CAD build for the part. Positions are in the model's coordinates, mm. A direction names the side the tool comes from. Round coordinates to 2 decimals unless told otherwise and drop trailing zeros. Loops run counter-clockwise (first coordinate to the right, second up) from the corner with the lowest first, then second, coordinate; pieces in that order, holes last. Notation, with made-up numbers: M -10.5,-18 L 31.5,-18 A19 cw 31.5,6 Z; hole C 3,72.25 d1. An arc over 180 degrees is marked long. Use one line per item in the form item = value.
from build123d import *

# Parameters (mm, degrees)
SKETCH1_W           = 25
SKETCH1_H           = 30
BOSS_EXTRUDE1_DEPTH = 12
BOSS_EXTRUDE6_DEPTH = 12
CHAMFER1_SIZE       = 7
CHAMFER1_SIZE2      = 12.124355653
BOSS_EXTRUDE4_DEPTH = 12
SKETCH7_R           = 2.8
CUT_EXTRUDE2_DEPTH  = 12
CHAMFER2_SIZE       = 8
CHAMFER2_SIZE_2     = 14
CHAMFER3_SIZE       = 14
CHAMFER3_SIZE_2     = 8
FILLET2_R           = 20
FILLET3_R           = 1
FILLET4_R           = 1.5
SKETCH10_R          = 1
CUT_EXTRUDE3_DEPTH  = 41.859515416
SKETCH11_R          = 2
CUT_EXTRUDE4_DEPTH  = 41.859515416
SKETCH12_R          = 3.5
BOSS_EXTRUDE8_DEPTH = 2
FILLET5_R           = 3


with BuildPart() as part:
    # Sketch1 → Boss-Extrude1 (new body)
    with BuildSketch(Plane(origin=(0, 0, 0), x_dir=(1, 0, 0), z_dir=(0, 1, 0))):
        Rectangle(SKETCH1_W, SKETCH1_H)
        Polygon((3.233161507, -5.6), (6.466323015, 0), (3.233161507, 5.6), (-3.233161507, 5.6), (-6.466323015, 0), (-3.233161507, -5.6), align=None, mode=Mode.SUBTRACT)
    extrude(amount=BOSS_EXTRUDE1_DEPTH)

    # Sketch8 → Boss-Extrude6 (add)
    with BuildSketch(Plane(origin=(0, 0, 0), x_dir=(1, 0, 0), z_dir=(0, 1, 0))):
        with BuildLine():
            Line((-4.5, -15), (4.5, -15))
            Line((4.5, -15), (4.5, -29))
            Line((4.5, -29), (1.7, -29))
            Line((1.7, -29), (1.7, -24))
            ThreePointArc((1.7, -24), (0, -22.3), (-1.7, -24))
            Line((-1.7, -24), (-1.7, -29))
            Line((-1.7, -29), (-4.5, -29))
            Line((-4.5, -29), (-4.5, -15))
        make_face()
    extrude(amount=BOSS_EXTRUDE6_DEPTH)

    # Chamfer1
    chamfer1_edges = [part.edges().sort_by_distance(p)[0] for p in [
        (-12.5, 6, -15),
        (12.5, 6, -15),
    ]]
    chamfer1_side = [part.faces().sort_by_distance(p)[0] for p in [
        (0, 6, -15),
    ]]
    chamfer(chamfer1_edges, length=CHAMFER1_SIZE, length2=CHAMFER1_SIZE2, reference=chamfer1_side[0])

    # Sketch6 → Boss-Extrude4 (add)
    with BuildSketch(Plane(origin=(0, 0, 0), x_dir=(1, 0, 0), z_dir=(0, 1, 0))):
        Polygon((-26.162950904, 6.363961031), (-12.5, -7.298989873), (-12.5, 2.875644347), (-11.047793697, 5.390939447), (-19.091883092, 13.435028843), align=None)
    extrude(amount=BOSS_EXTRUDE4_DEPTH)

    # Sketch7 → Cut-Extrude2 (cut)
    with BuildSketch(Plane(origin=(-9.899494937, 0, 9.899494937), x_dir=(0.7071067811865438, 0, 0.7071067811865512), z_dir=(-0.7071067811865512, 0, 0.7071067811865438))):
        with Locations((-18, 6)):
            Circle(SKETCH7_R)
    extrude(amount=-CUT_EXTRUDE2_DEPTH, mode=Mode.SUBTRACT)

    # Chamfer2
    # the kernel refuses this chamfer: 14, 8 mm, written as the material it adds along each edge
    with BuildSketch(Plane(origin=(4.5, 0, 15), x_dir=(0.9982794274996464, 0, -0.05863603525971087), z_dir=(0, 1, 0))) as chamfer2_piece_1:
        Polygon((CHAMFER2_SIZE * 0.9982794275, -CHAMFER2_SIZE * 0.0586360352597), (-CHAMFER2_SIZE_2 * 0.0586360352597, -CHAMFER2_SIZE_2 * 0.9982794275), (0, 0), align=None)
    extrude(amount=12)

    # Chamfer3
    # the kernel refuses this chamfer: 14, 8 mm, written as the material it adds along each edge
    with BuildSketch(Plane(origin=(-4.5, 0, 15), x_dir=(0.019175933519162247, 0, 0.9998161248818048), z_dir=(0, 1, 0))) as chamfer3_piece_1:
        Polygon((CHAMFER3_SIZE * 0.999816124882, -CHAMFER3_SIZE * 0.0191759335192), (-CHAMFER3_SIZE_2 * 0.0191759335192, -CHAMFER3_SIZE_2 * 0.999816124882), (0, 0), align=None)
    extrude(amount=12)

    # Fillet2
    fillet2_edges = [part.edges().sort_by_distance(p)[0] for p in [
        (12.5, 6, 15),
        (-12.5, 6, 15),
    ]]
    fillet(fillet2_edges, radius=FILLET2_R)

    # Fillet3
    fillet3_edges = [part.edges().sort_by_distance(p)[0] for p in [
        (-4.5, 6, 29),
        (-1.7, 6, 29),
        (1.7, 6, 29),
        (4.5, 6, 29),
    ]]
    fillet(fillet3_edges, radius=FILLET3_R)

    # Fillet4
    fillet4_edges = [part.edges().sort_by_distance(p)[0] for p in [
        (-12.5, 6, 7.298989873),
        (-11.047793697, 6, -5.390939447),
    ]]
    fillet(fillet4_edges, radius=FILLET4_R)

    # Sketch10 → Cut-Extrude3 (cut, through all)
    with BuildSketch(Plane(origin=(0, 12, 0), x_dir=(1, 0, 0), z_dir=(0, 1, 0))):
        with Locations(Location((0, -13, 0), (0, 0, 270))):
            Circle(SKETCH10_R)
    extrude(amount=-CUT_EXTRUDE3_DEPTH, mode=Mode.SUBTRACT)

    # Sketch11 → Cut-Extrude4 (cut, through all)
    with BuildSketch(Plane(origin=(0, 0, 0), x_dir=(0, 0, -1), z_dir=(1, 0, 0))):
        with Locations((-13, 6)):
            Circle(SKETCH11_R)
    extrude(amount=-CUT_EXTRUDE4_DEPTH, mode=Mode.SUBTRACT)

    # Sketch12 → Boss-Extrude8 (add)
    with BuildSketch(Plane(origin=(0, 12, 0), x_dir=(1, 0, 0), z_dir=(0, 1, 0))):
        Polygon((3.233161507, 5.6), (-3.233161507, 5.6), (-6.466323015, 0), (-3.233161507, -5.6), (3.233161507, -5.6), (6.466323015, 0), align=None)
        with Locations(Location((0, 0, 0), (0, 0, 270))):
            Circle(SKETCH12_R, mode=Mode.SUBTRACT)
    extrude(amount=-BOSS_EXTRUDE8_DEPTH)

    # Fillet5
    # the kernel refuses this fillet: 3 mm, written as the material it takes off along each edge
    with BuildSketch(Plane(origin=(-19.091883092, -7.5, -13.435028843), x_dir=(-0.7071067811865517, 0, 0.7071067811865434), z_dir=(0, 1, 0))) as fillet5_piece_1:
        with BuildLine():
            CenterArc((FILLET5_R, FILLET5_R), FILLET5_R, 180, 90)
            Line((0, FILLET5_R), (0, 0))
            Line((0, 0), (FILLET5_R, 0))
        make_face()
    extrude(amount=27, mode=Mode.SUBTRACT)


solid = part.part
1. Cut at C-C on y = 2.5. State how many separate pieces and enclosed holes the cut face has, and give its area (3 significant figures).
Completed:
separate_pieces = 1
enclosed_holes = 2
area = 910 mm2
2. Drop flat-ended pins along their axis: P1, Ø1, axis at y = 9, z = 17, coming from the -X side; P2, Ø1.2, axis at x = 0, z = 13, coming from the -Y side; P3, Ø3, axis at y = 8.5, z = 27, coming from the -X side; P4, Ø2, axis at y = 4.5, z = -3.5, coming from the +X side. Give the stop position or say it passes through.
Completed:
P1 = -11.3
P2 = through
P3 = -6.5
P4 = 12.5
3. Probe line 1 along Z through (x, y) = (-6, 6.5) (1 decimal); line 2 along Y through (x, z) = (-3, 13); line 3 along Z through (x, y) = (-4.5, 6). List the from-to ranges inside material, lowest first. Write a range as from..to.
Completed:
line_1 = -14.1..-0.8, 0.8..11.1, 14.9..26.4
line_2 = 0..4, 8..12
line_3 = -15..-3.41, 3.41..11, 15..28.81
4. Cut at B-B on z = 13.5. Write the cut outline in (x, y), and give its area (3 significant figures).
Completed:
outline = M -12.13,0 L -0.87,0 L -0.87,4.06 L -12.13,4.06 Z; M -12.13,7.94 L -0.87,7.94 L -0.87,12 L -12.13,12 Z; M 0.87,0 L 12.13,0 L 12.13,12 L 0.87,12 Z
area = 227 mm2
5. Pull direction Y, two halves, no side cores. Call faces 1 (the face through (0, 6, 14.4)), 2 (the face through (0, 5, -5.6)), 3 (the face through (-19.571, 3.267, -6.744)), 4 (the face through (-2, 0, 7)): +Y half, -Y half, draft (parallel to the pull), parting line (faces both ways), or undercut.
Completed:
face_1 = undercut
face_2 = draft
face_3 = undercut
face_4 = -Y half
6. Tool access for faces 5 (the face through (-12.5, 6, 9)), 6 (the face through (-13.66, 4.583, -8.003)), 7 (the face through (1.985, 6.084, 28.699)): list every direction of +Z, -Z, +X, -X, +Y, -Y with a clear straight run to the whole face (end or side of a thin tool).
Completed:
face_5 = +Z, -X, +Y, -Y
face_6 = -Z, +Y, -Y
face_7 = +Z, +Y, -Y
7. Cut at A-A on y = 11. Write the cut outline in (x, z), and give its area (3 significant figures).
Completed:
outline = M -26.16,-6.36 L -21.21,-11.31 A3 ccw -16.97,-11.31 L -12.43,-6.77 A1.5 cw -10.07,-7.08 L -5.5,-15 L 5.5,-15 L 12.5,-2.88 L 12.5,9.69 A20 ccw 9.86,19.61 L 4.79,28.5 A1 ccw 3.92,29 L 2.7,29 A1 ccw 1.7,28 L 1.7,24 A1.7 cw -1.7,24 L -1.7,28 A1 ccw -2.7,29 L -3.92,29 A1 ccw -4.79,28.5 L -9.86,19.61 A20 ccw -12.5,9.69 L -12.5,7.92 A1.5 cw -12.94,6.86 Z; hole C 0,0 d7; hole C 0,13 d2
area = 980 mm2
